Geometry check sheet. Reference: the model listing, model coordinates, mm. A direction names the side the tool comes from. Round coordinates to 2 decimals unless told otherwise and drop trailing zeros. Put each result on its own line as item: value. Start each with the question number.
(1) Gauge pin test, flat ends, axial feed: pin 1 (1.9 mm diameter, centred on x = 71.5, z = -1.5, fed in from -Y); pin 2 (1 mm diameter, centred on y = 2.5, z = 2, fed in from +X); pin 3 (4 mm diameter, centred on y = 4, z = -3, fed in from +X). Record the tip position at first contact, or that the pin passes through.
(2) Material ranges on probe 1 along Y at (x, z) = (16, 3); probe 2 along Z at (x, y) = (2.5, 7) (3 decimals); probe 3 along Z at (x, y) = (79, 2), recorded low to high.
(3) Tool access check on faces 1 (the cylindrical face through (26.98, 0.62, 0.94)), 2 (the flat face through (66, 6.45, -2)), 3 (the flat face through (108, 0, 0)). Record the directions out of +Z, -Z, +X, -X, +Y, -Y that give a thin tool (end or side, any length) a straight path to the whole face; none if there is none.
(4) Mould release check, pull along Z, two halves, no side actions. Record for faces 4 (the flat face through (114, 6.45, -2)), 5 (the flat face through (28, 0, 0)), 6 (the cylindrical face through (109.804, 3.689, 1.142)): pulls with the +Z half, pulls with the -Z half, needs draft (parallel to the pull), parting line crosses it, or undercut.
(5) Section check A-A on y = 2.25. Count the separate pieces of the cut face and the enclosed holes in it, then the cut area to 3 significant figures.
from build123d import *

# Parameters (mm, degrees)
BOSS_EXTRUDE1_DEPTH        = 7.3
SKETCH2_R                  = 2.475
CUT_EXTRUDE1_DEPTH         = 117.195137592
SKETCH3_R                  = 3.125
CUT_EXTRUDE2_DEPTH         = 0.85
LPATTERN1_COUNT            = 15
LPATTERN1_PITCH            = 8
LPATTERN1_COPY_1_SKETCH_R  = 3.125
LPATTERN1_COPY_1_DEPTH     = 0.85
LPATTERN1_COPY_2_SKETCH_R  = 3.125
LPATTERN1_COPY_2_DEPTH     = 0.85
LPATTERN1_COPY_3_SKETCH_R  = 3.125
LPATTERN1_COPY_3_DEPTH     = 0.85
LPATTERN1_COPY_4_SKETCH_R  = 3.125
LPATTERN1_COPY_4_DEPTH     = 0.85
LPATTERN1_COPY_5_SKETCH_R  = 3.125
LPATTERN1_COPY_5_DEPTH     = 0.85
LPATTERN1_COPY_6_SKETCH_R  = 3.125
LPATTERN1_COPY_6_DEPTH     = 0.85
LPATTERN1_COPY_7_SKETCH_R  = 3.125
LPATTERN1_COPY_7_DEPTH     = 0.85
LPATTERN1_COPY_8_SKETCH_R  = 3.125
LPATTERN1_COPY_8_DEPTH     = 0.85
LPATTERN1_COPY_9_SKETCH_R  = 3.125
LPATTERN1_COPY_9_DEPTH     = 0.85
LPATTERN1_COPY_10_SKETCH_R = 3.125
LPATTERN1_COPY_10_DEPTH    = 0.85
LPATTERN1_COPY_11_SKETCH_R = 3.125
LPATTERN1_COPY_11_DEPTH    = 0.85
LPATTERN1_COPY_12_SKETCH_R = 3.125
LPATTERN1_COPY_12_DEPTH    = 0.85
LPATTERN1_COPY_13_SKETCH_R = 3.125
LPATTERN1_COPY_13_DEPTH    = 0.85
LPATTERN1_COPY_14_SKETCH_R = 3.125
LPATTERN1_COPY_14_DEPTH    = 0.85
CHAMFER1_SIZE              = 0.4


with BuildPart() as part:
    # Sketch1 → Boss-Extrude1 (new body)
    with BuildSketch(Plane(origin=(0, 0, 0), x_dir=(1, 0, 0), z_dir=(0, 1, 0))):
        with BuildLine():
            Line((0, 3.9), (112, 3.9))
            ThreePointArc((112, 3.9), (115.9, 0), (112, -3.9))
            Line((112, -3.9), (0, -3.9))
            ThreePointArc((0, -3.9), (-3.9, 0), (0, 3.9))
        make_face()
    extrude(amount=BOSS_EXTRUDE1_DEPTH)

    # Sketch2 → Cut-Extrude1 (cut, through all)
    with BuildSketch(Plane(origin=(0, 7.3, 0), x_dir=(1, 0, 0), z_dir=(0, 1, 0))):
        with Locations(Location((0, 0, 0), (0, 0, 270))):
            Circle(SKETCH2_R)
    cut_extrude1 = extrude(amount=-CUT_EXTRUDE1_DEPTH, mode=Mode.SUBTRACT)

    # Sketch3 → Cut-Extrude2 (cut)
    with BuildSketch(Plane(origin=(0, 7.3, 0), x_dir=(1, 0, 0), z_dir=(0, 1, 0))):
        with Locations(Location((0, 0, 0), (0, 0, 270))):
            Circle(SKETCH3_R)
    cut_extrude2 = extrude(amount=-CUT_EXTRUDE2_DEPTH, mode=Mode.SUBTRACT)

    # Mirror1: Cut-Extrude2 across plane
    add(cut_extrude2.mirror(Plane.ZX.offset(3.65)), mode=Mode.SUBTRACT)

    # LPattern1: Cut-Extrude1, Cut-Extrude2 ×15
    with Locations(*[(i * LPATTERN1_PITCH, 0, 0) for i in range(1, LPATTERN1_COUNT)]):
        add(cut_extrude1, mode=Mode.SUBTRACT)
        add(cut_extrude2, mode=Mode.SUBTRACT)

    # LPattern1 copy 1 sketch → LPattern1 copy 1 (cut)
    with BuildSketch(Plane(origin=(8, 0, 0), x_dir=(1, 0, 0), z_dir=(0, -1, 0))):
        Circle(LPATTERN1_COPY_1_SKETCH_R)
    extrude(amount=-LPATTERN1_COPY_1_DEPTH, mode=Mode.SUBTRACT)

    # LPattern1 copy 2 sketch → LPattern1 copy 2 (cut)
    with BuildSketch(Plane(origin=(16, 0, 0), x_dir=(1, 0, 0), z_dir=(0, -1, 0))):
        Circle(LPATTERN1_COPY_2_SKETCH_R)
    extrude(amount=-LPATTERN1_COPY_2_DEPTH, mode=Mode.SUBTRACT)

    # LPattern1 copy 3 sketch → LPattern1 copy 3 (cut)
    with BuildSketch(Plane(origin=(24, 0, 0), x_dir=(1, 0, 0), z_dir=(0, -1, 0))):
        Circle(LPATTERN1_COPY_3_SKETCH_R)
    extrude(amount=-LPATTERN1_COPY_3_DEPTH, mode=Mode.SUBTRACT)

    # LPattern1 copy 4 sketch → LPattern1 copy 4 (cut)
    with BuildSketch(Plane(origin=(32, 0, 0), x_dir=(1, 0, 0), z_dir=(0, -1, 0))):
        Circle(LPATTERN1_COPY_4_SKETCH_R)
    extrude(amount=-LPATTERN1_COPY_4_DEPTH, mode=Mode.SUBTRACT)

    # LPattern1 copy 5 sketch → LPattern1 copy 5 (cut)
    with BuildSketch(Plane(origin=(40, 0, 0), x_dir=(1, 0, 0), z_dir=(0, -1, 0))):
        Circle(LPATTERN1_COPY_5_SKETCH_R)
    extrude(amount=-LPATTERN1_COPY_5_DEPTH, mode=Mode.SUBTRACT)

    # LPattern1 copy 6 sketch → LPattern1 copy 6 (cut)
    with BuildSketch(Plane(origin=(48, 0, 0), x_dir=(1, 0, 0), z_dir=(0, -1, 0))):
        Circle(LPATTERN1_COPY_6_SKETCH_R)
    extrude(amount=-LPATTERN1_COPY_6_DEPTH, mode=Mode.SUBTRACT)

    # LPattern1 copy 7 sketch → LPattern1 copy 7 (cut)
    with BuildSketch(Plane(origin=(56, 0, 0), x_dir=(1, 0, 0), z_dir=(0, -1, 0))):
        Circle(LPATTERN1_COPY_7_SKETCH_R)
    extrude(amount=-LPATTERN1_COPY_7_DEPTH, mode=Mode.SUBTRACT)

    # LPattern1 copy 8 sketch → LPattern1 copy 8 (cut)
    with BuildSketch(Plane(origin=(64, 0, 0), x_dir=(1, 0, 0), z_dir=(0, -1, 0))):
        Circle(LPATTERN1_COPY_8_SKETCH_R)
    extrude(amount=-LPATTERN1_COPY_8_DEPTH, mode=Mode.SUBTRACT)

    # LPattern1 copy 9 sketch → LPattern1 copy 9 (cut)
    with BuildSketch(Plane(origin=(72, 0, 0), x_dir=(1, 0, 0), z_dir=(0, -1, 0))):
        Circle(LPATTERN1_COPY_9_SKETCH_R)
    extrude(amount=-LPATTERN1_COPY_9_DEPTH, mode=Mode.SUBTRACT)

    # LPattern1 copy 10 sketch → LPattern1 copy 10 (cut)
    with BuildSketch(Plane(origin=(80, 0, 0), x_dir=(1, 0, 0), z_dir=(0, -1, 0))):
        Circle(LPATTERN1_COPY_10_SKETCH_R)
    extrude(amount=-LPATTERN1_COPY_10_DEPTH, mode=Mode.SUBTRACT)

    # LPattern1 copy 11 sketch → LPattern1 copy 11 (cut)
    with BuildSketch(Plane(origin=(88, 0, 0), x_dir=(1, 0, 0), z_dir=(0, -1, 0))):
        Circle(LPATTERN1_COPY_11_SKETCH_R)
    extrude(amount=-LPATTERN1_COPY_11_DEPTH, mode=Mode.SUBTRACT)

    # LPattern1 copy 12 sketch → LPattern1 copy 12 (cut)
    with BuildSketch(Plane(origin=(96, 0, 0), x_dir=(1, 0, 0), z_dir=(0, -1, 0))):
        Circle(LPATTERN1_COPY_12_SKETCH_R)
    extrude(amount=-LPATTERN1_COPY_12_DEPTH, mode=Mode.SUBTRACT)

    # LPattern1 copy 13 sketch → LPattern1 copy 13 (cut)
    with BuildSketch(Plane(origin=(104, 0, 0), x_dir=(1, 0, 0), z_dir=(0, -1, 0))):
        Circle(LPATTERN1_COPY_13_SKETCH_R)
    extrude(amount=-LPATTERN1_COPY_13_DEPTH, mode=Mode.SUBTRACT)

    # LPattern1 copy 14 sketch → LPattern1 copy 14 (cut)
    with BuildSketch(Plane(origin=(112, 0, 0), x_dir=(1, 0, 0), z_dir=(0, -1, 0))):
        Circle(LPATTERN1_COPY_14_SKETCH_R)
    extrude(amount=-LPATTERN1_COPY_14_DEPTH, mode=Mode.SUBTRACT)

    # Chamfer1
    # the kernel refuses this chamfer: 0.4 mm, written as the material it takes off along each edge
    with BuildSketch(Plane(origin=(8, 0, 0), x_dir=(1, 0, 0), z_dir=(0, 0, -1))) as chamfer1_piece_1:
        Polygon((3.125 + CHAMFER1_SIZE, 0), (3.125, -CHAMFER1_SIZE), (3.125, 0), align=None)
    revolve(axis=Axis((8, 0, 0), (0, -1, 0)), mode=Mode.SUBTRACT)
    with BuildSketch(Plane(origin=(16, 0, 0), x_dir=(1, 0, 0), z_dir=(0, 0, -1))) as chamfer1_piece_2:
        Polygon((3.125 + CHAMFER1_SIZE, 0), (3.125, -CHAMFER1_SIZE), (3.125, 0), align=None)
    revolve(axis=Axis((16, 0, 0), (0, -1, 0)), mode=Mode.SUBTRACT)
    with BuildSketch(Plane(origin=(24, 0, 0), x_dir=(1, 0, 0), z_dir=(0, 0, -1))) as chamfer1_piece_3:
        Polygon((3.125 + CHAMFER1_SIZE, 0), (3.125, -CHAMFER1_SIZE), (3.125, 0), align=None)
    revolve(axis=Axis((24, 0, 0), (0, -1, 0)), mode=Mode.SUBTRACT)
    with BuildSketch(Plane(origin=(32, 0, 0), x_dir=(1, 0, 0), z_dir=(0, 0, -1))) as chamfer1_piece_4:
        Polygon((3.125 + CHAMFER1_SIZE, 0), (3.125, -CHAMFER1_SIZE), (3.125, 0), align=None)
    revolve(axis=Axis((32, 0, 0), (0, -1, 0)), mode=Mode.SUBTRACT)
    with BuildSketch(Plane(origin=(40, 0, 0), x_dir=(1, 0, 0), z_dir=(0, 0, -1))) as chamfer1_piece_5:
        Polygon((3.125 + CHAMFER1_SIZE, 0), (3.125, -CHAMFER1_SIZE), (3.125, 0), align=None)
    revolve(axis=Axis((40, 0, 0), (0, -1, 0)), mode=Mode.SUBTRACT)
    with BuildSketch(Plane(origin=(48, 0, 0), x_dir=(1, 0, 0), z_dir=(0, 0, -1))) as chamfer1_piece_6:
        Polygon((3.125 + CHAMFER1_SIZE, 0), (3.125, -CHAMFER1_SIZE), (3.125, 0), align=None)
    revolve(axis=Axis((48, 0, 0), (0, -1, 0)), mode=Mode.SUBTRACT)
    with BuildSketch(Plane(origin=(56, 0, 0), x_dir=(1, 0, 0), z_dir=(0, 0, -1))) as chamfer1_piece_7:
        Polygon((3.125 + CHAMFER1_SIZE, 0), (3.125, -CHAMFER1_SIZE), (3.125, 0), align=None)
    revolve(axis=Axis((56, 0, 0), (0, -1, 0)), mode=Mode.SUBTRACT)
    with BuildSketch(Plane(origin=(64, 0, 0), x_dir=(1, 0, 0), z_dir=(0, 0, -1))) as chamfer1_piece_8:
        Polygon((3.125 + CHAMFER1_SIZE, 0), (3.125, -CHAMFER1_SIZE), (3.125, 0), align=None)
    revolve(axis=Axis((64, 0, 0), (0, -1, 0)), mode=Mode.SUBTRACT)
    with BuildSketch(Plane(origin=(72, 0, 0), x_dir=(1, 0, 0), z_dir=(0, 0, -1))) as chamfer1_piece_9:
        Polygon((3.125 + CHAMFER1_SIZE, 0), (3.125, -CHAMFER1_SIZE), (3.125, 0), align=None)
    revolve(axis=Axis((72, 0, 0), (0, -1, 0)), mode=Mode.SUBTRACT)
    with BuildSketch(Plane(origin=(80, 0, 0), x_dir=(1, 0, 0), z_dir=(0, 0, -1))) as chamfer1_piece_10:
        Polygon((3.125 + CHAMFER1_SIZE, 0), (3.125, -CHAMFER1_SIZE), (3.125, 0), align=None)
    revolve(axis=Axis((80, 0, 0), (0, -1, 0)), mode=Mode.SUBTRACT)
    with BuildSketch(Plane(origin=(88, 0, 0), x_dir=(1, 0, 0), z_dir=(0, 0, -1))) as chamfer1_piece_11:
        Polygon((3.125 + CHAMFER1_SIZE, 0), (3.125, -CHAMFER1_SIZE), (3.125, 0), align=None)
    revolve(axis=Axis((88, 0, 0), (0, -1, 0)), mode=Mode.SUBTRACT)
    with BuildSketch(Plane(origin=(96, 0, 0), x_dir=(1, 0, 0), z_dir=(0, 0, -1))) as chamfer1_piece_12:
        Polygon((3.125 + CHAMFER1_SIZE, 0), (3.125, -CHAMFER1_SIZE), (3.125, 0), align=None)
    revolve(axis=Axis((96, 0, 0), (0, -1, 0)), mode=Mode.SUBTRACT)
    with BuildSketch(Plane(origin=(104, 0, 0), x_dir=(1, 0, 0), z_dir=(0, 0, -1))) as chamfer1_piece_13:
        Polygon((3.125 + CHAMFER1_SIZE, 0), (3.125, -CHAMFER1_SIZE), (3.125, 0), align=None)
    revolve(axis=Axis((104, 0, 0), (0, -1, 0)), mode=Mode.SUBTRACT)
    with BuildSketch(Plane(origin=(112, 0, 0), x_dir=(1, 0, 0), z_dir=(0, 0, -1))) as chamfer1_piece_14:
        Polygon((3.125 + CHAMFER1_SIZE, 0), (3.125, -CHAMFER1_SIZE), (3.125, 0), align=None)
    revolve(axis=Axis((112, 0, 0), (0, -1, 0)), mode=Mode.SUBTRACT)
    with BuildSketch(Plane(origin=(0, 0, 0), x_dir=(0, 0, 1), z_dir=(-1, 0, 0))) as chamfer1_piece_15:
        Polygon((3.125 + CHAMFER1_SIZE, 0), (3.125, CHAMFER1_SIZE), (3.125, 0), align=None)
    revolve(axis=Axis((0, 0, 0), (0, 1, 0)), mode=Mode.SUBTRACT)
    with BuildSketch(Plane(origin=(0, 0, -3.9), x_dir=(0, -0.027495876610586386, 0.9996219169112968), z_dir=(1, 0, 0))) as chamfer1_piece_16:
        Polygon((CHAMFER1_SIZE * 0.999621916911, -CHAMFER1_SIZE * 0.0274958766106), (-CHAMFER1_SIZE * 0.0274958766106, -CHAMFER1_SIZE * 0.999621916911), (0, 0), align=None)
    extrude(amount=112, mode=Mode.SUBTRACT)
    with BuildSketch(Plane(origin=(112, 0, 0), x_dir=(0, 0, -1), z_dir=(-1, 0, 0))) as chamfer1_piece_17:
        Polygon((3.9, -CHAMFER1_SIZE), (3.9 - CHAMFER1_SIZE, 0), (3.9, 0), align=None)
    revolve(axis=Axis((112, 0, 0), (0, -1, 0)), revolution_arc=180, mode=Mode.SUBTRACT)
    with BuildSketch(Plane(origin=(112, 0, 3.9), x_dir=(0, 0.9996219169112968, 0.027495876610586275), z_dir=(-1, 0, 0))) as chamfer1_piece_18:
        Polygon((CHAMFER1_SIZE * 0.999621916911, CHAMFER1_SIZE * 0.0274958766106), (-CHAMFER1_SIZE * 0.0274958766106, CHAMFER1_SIZE * 0.999621916911), (0, 0), align=None)
    extrude(amount=112, mode=Mode.SUBTRACT)
    with BuildSketch(Plane(origin=(0, 0, 0), x_dir=(0, 0, 1), z_dir=(1, 0, 0))) as chamfer1_piece_19:
        Polygon((3.9, -CHAMFER1_SIZE), (3.9 - CHAMFER1_SIZE, 0), (3.9, 0), align=None)
    revolve(axis=Axis((0, 0, 0), (0, -1, 0)), revolution_arc=180, mode=Mode.SUBTRACT)


solid = part.part
Answers follow:
1. pin 1: stops at y = 0.85
1. pin 2: stops at x = 115.6
1. pin 3: stops at x = 115.77
2. probe 1: y = 0.85 to 6.45
2. probe 2: z = -3.9 to -1.875, 1.875 to 3.9
2. probe 3: z = -3.9 to -2.26, 2.26 to 3.9
3. face 1: -Y
3. face 2: +Y
3. face 3: +Z, -Z, +X, -X, -Y
4. face 4: undercut
4. face 5: needs draft
4. face 6: undercut
5. separate pieces: 1
5. enclosed holes: 15
5. area: 633 mm^2
